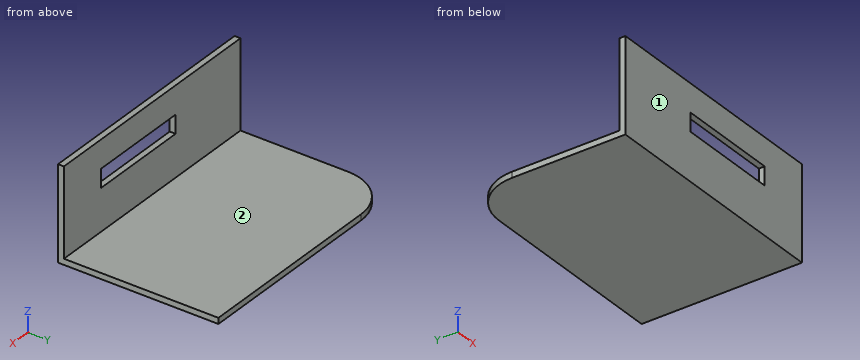
```python
from build123d import *

# Parameters (mm, degrees)
F0_W      = 52.705
F0_H      = 34.7472
F0_W_2    = 50.165
F0_H_2    = 32.2072
F1_DEPTH  = 20.32
F2_DEPTH  = 1.27
F3_R      = 10.16
F6_W      = 22.0472
F6_H      = 1.27
F7_DEPTH  = 0.381
F8_W      = 33.4772
F8_H      = 19.05
F9_DEPTH  = 78.74
F10_W     = 22.225
F10_H     = 3.96875
F11_DEPTH = 25.4


with BuildPart() as f1:
    # F0 (on Top) → F1 (new body)
    with BuildSketch(Plane.XY):
        with Locations((-38.596277, 2.575059)):
            Rectangle(F0_W, F0_H)
        with Locations((-38.596277, 2.575059)):
            Rectangle(F0_W_2, F0_H_2, mode=Mode.SUBTRACT)
    extrude(amount=F1_DEPTH)

    # F0 (on Top) → F2 (join)
    with BuildSketch(Plane.XY):
        with Locations((-38.596277, 2.575059)):
            Rectangle(F0_W_2, F0_H_2)
    extrude(amount=F2_DEPTH)

    # F3
    f3_edges = [f1.edges().sort_by_distance(p)[0] for p in [
        (-64.948777, 19.948659, 10.16),
        (-63.678777, 18.678659, 10.795),
    ]]
    fillet(f3_edges, radius=F3_R)

    # F6 (on face) → F7 (join)
    with BuildSketch(Plane(origin=(-13.513777, 0, 0), x_dir=(0, -1, 0), z_dir=(-1, 0, 0))):
        with Locations((2.504941, 8.5725)):
            Rectangle(F6_W, F6_H)
    extrude(amount=F7_DEPTH)

    # F8 (on face) → F9 (cut)
    with BuildSketch(Plane.YZ.offset(-12.243777)):
        with Locations((3.210059, 10.795)):
            Rectangle(F8_W, F8_H)
    extrude(amount=-F9_DEPTH, mode=Mode.SUBTRACT)

    # F10 (on face) → F11 (cut)
    with BuildSketch(Plane.XZ.offset(14.798541)):
        with Locations((-34.468777, 12.303125)):
            Rectangle(F10_W, F10_H)
    extrude(amount=-F11_DEPTH, mode=Mode.SUBTRACT)


solid = f1.part
```
Build history of the part. All positions in model axes, mm. Face numbers are marked on the shaded views. A direction names the side the tool comes from. Round coordinates to 2 decimals unless told otherwise and drop trailing zeros. Order: outer loops, then holes, each group sorted by start corner. A loop starts at its lowest first (then second) coordinate and runs counter-clockwise, first axis right, second up. Notation, with made-up numbers: (57, 70.25) -> (90, 70.25) arc R27 cw to (90, 97.25) -> close; hole circle Ø4 at (34.25, 40.25). An arc over 180 degrees is marked (long way). Answer in a Markdown table with one row per item.
1) Band-saw the part on D-D on y = -6.5. Give the cut face in (x, z).
Values:
| item | result |
|---|---|
| outline | (-64.95, 0) -> (-12.24, 0) -> (-12.24, 1.27) -> (-64.95, 1.27) -> close |
2) Band-saw the part on C-C on x = -20.5. Give the cut face in (y, z), and give its area (3 significant figures).
Values:
| item | result |
|---|---|
| outline | (-14.8, 0) -> (19.95, 0) -> (19.95, 1.27) -> (-13.53, 1.27) -> (-13.53, 20.32) -> (-14.8, 20.32) -> close |
| area | 68.3 mm2 |
3) Band-saw the part on B-B on z = 12. Give the cut face in (x, y), and give its area (3 significant figures).
Values:
| item | result |
|---|---|
| outline | (-64.95, -14.8) -> (-45.58, -14.8) -> (-45.58, -13.53) -> (-64.95, -13.53) -> close; (-23.36, -14.8) -> (-12.24, -14.8) -> (-12.24, -13.53) -> (-23.36, -13.53) -> close |
| area | 38.7 mm2 |
4) Which spindle directions (+Z, -Z, +X, -X, +Y, -Y) get a long thin tool onto all of the face, cutting with end or side? Do the marked faces 1 and 2. Say none if no direction does.
Values:
| item | result |
|---|---|
| face 1 | +Z, -Z, +X, -X, -Y |
| face 2 | +Z, +X, -X, +Y |
5) Pin check, flat tips, straight feed: P1, Ø8, axis at x = -27, y = 7, coming from the +Z side; P2, Ø8, axis at x = -52, z = 8.5, coming from the +Y side; P3, Ø1.5, axis at y = 6, z = 4, coming from the +X side. Stop position of each tip, or through.
Values:
| item | result |
|---|---|
| P1 | z = 1.27 |
| P2 | y = -13.53 |
| P3 | through |
6) Band-saw the part on A-A on x = -42.5. Give the cut face in (y, z).
Values:
| item | result |
|---|---|
| outline | (-14.8, 0) -> (19.95, 0) -> (19.95, 1.27) -> (-13.53, 1.27) -> (-13.53, 10.32) -> (-14.8, 10.32) -> close; (-14.8, 14.29) -> (-13.53, 14.29) -> (-13.53, 20.32) -> (-14.8, 20.32) -> close |
7) Wall check: L1, parallel to Z at x = -53.5, y = -11; L2, parallel to Y at x = -57, z = 9.75. Give the ranges that are in metal, low to high.
Values:
| item | result |
|---|---|
| L1 | 0 to 1.27 |
| L2 | -14.8 to -13.53 |
